```python
from build123d import *

# Parameters (mm, degrees)
SKETCH_1_R      = 25
EXTRUDE_1_DEPTH = 5
EXTRUDE_2_DEPTH = 5


with BuildPart() as part:
    # 草图1 → 凸台-拉伸1 (new body)
    with BuildSketch(Plane(origin=(0, 0, 0), x_dir=(1, 0, 0), z_dir=(0, 1, 0))):
        with Locations(Location((0, 0, 0), (0, 0, 270))):
            Circle(SKETCH_1_R)
    extrude(amount=EXTRUDE_1_DEPTH)

    # 草图2 → 凸台-拉伸2 (add)
    with BuildSketch(Plane.XY.offset(5)):
        with BuildLine():
            Line((5.875511267, 5), (15.054948865, 19.8740887))
            ThreePointArc((15.054948865, 19.8740887), (13.4259113, 26.754948865), (6.545051135, 25.1259113))
            Line((6.545051135, 25.1259113), (-5.875511267, 5))
            Line((-5.875511267, 5), (5.875511267, 5))
        make_face()
    extrude(amount=EXTRUDE_2_DEPTH)


solid = part.part
```
Verification items for the finished model (mm, model axes). A direction names the side the tool comes from. Coordinates: 2 decimals unless noted, no trailing zeros. Loops run counter-clockwise (first coordinate to the right, second up) from the corner with the lowest first, then second, coordinate; pieces in that order, holes last. Notation, with made-up numbers: (54.5, 51) - (93.5, 51) arc R14 ccw to (93.5, 72) - close; hole circle Ø11 at (20, 12.25). An arc over 180 degrees is marked (long way). Return JSON: item names as keys, results as strings.
1. Section check C-C, the plane z = 6. Record the boundary of the cut face in (x, y).
Established:
{"outline": "(-24.27, 0) - (24.27, 0) - (24.27, 5) - (5.88, 5) - (15.05, 19.87) arc R5 ccw to (6.55, 25.13) - (-5.88, 5) - (-24.27, 5) - close"}
2. Section check A-A, the plane x = 10.8. Record the boundary of the cut face in (y, z), then the cut area to 3 significant figures.
Established:
{"outline": "(0, -22.55) - (5, -22.55) - (5, 22.55) - (0, 22.55) - close; (12.98, 5) - (27.5, 5) - (27.5, 10) - (12.98, 10) - close", "area": "298 mm2"}
3. Section check D-D, the plane y = 22.5. Record the boundary of the cut face in (x, z).
Established:
{"outline": "(4.92, 5) - (15.8, 5) - (15.8, 10) - (4.92, 10) - close"}
4. Section check B-B, the plane x = 0. Record the boundary of the cut face in (y, z).
Established:
{"outline": "(0, -25) - (5, -25) - (5, 5) - (14.52, 5) - (14.52, 10) - (5, 10) - (5, 25) - (0, 25) - close"}
5. Go/stop test with flat-tipped pins: pin 1 (4 mm diameter, centred on x = 3, y = 23, fed in from -Z); pin 2 (3 mm diameter, centred on x = 6, z = 15, fed in from +Y); pin 3 (12 mm diameter, centred on y = 18, z = -4.5, fed in from +X); pin 4 (6.5 mm diameter, centred on x = 6, y = 20.5, fed in from +Z). Record where each tip stops, or that it passes through.
Established:
{"pin 1": "stops at z = 5", "pin 2": "stops at y = 5", "pin 3": "passes through", "pin 4": "stops at z = 10"}
6. Mould release check, pull along Y, two halves, no side actions. Record for faces 4 (the flat face through (10.4, 12.33, 7.46)), 5 (the cylindrical face through (7.509, 2.465, 23.846)), 6 (the flat face through (0, 0, 0)): +Y half, -Y half, draft (parallel to the pull), parting line (faces both ways), or undercut.
Established:
{"face 4": "undercut", "face 5": "draft", "face 6": "-Y half"}
7. Tool access check on faces 1 (the flat face through (7, 16, 10)), 2 (the cylindrical face through (13.519, 26.696, 7.465)), 3 (the flat face through (7, 16, 5)). Record the directions out of +Z, -Z, +X, -X, +Y, -Y that give a thin tool (end or side, any length) a straight path to the whole face; none if there is none.
Established:
{"face 1": "+Z, +X, -X, +Y", "face 2": "+Z, -Z", "face 3": "-Z, +X, -X, +Y"}
8. Thickness scan on L1, parallel to Y at x = -0.5, z = -11.5; L2, parallel to Z at x = 8.5, y = 17.5; L3, parallel to Y at x = 0, z = 8. Record the ranges inside material, lowest first.
Established:
{"L1": "y = 0 to 5", "L2": "z = 5 to 10", "L3": "y = 0 to 14.52"}
